Here's how the part is built. I have some questions about the finished solid (model axes, mm). A direction names the side the tool comes from. Give positions to 0.01 mm unless a question says otherwise; leave off trailing zeros. Write each loop counter-clockwise with the first axis right and the second up, starting at its lowest first coordinate (ties: lowest second). Pieces come first, ordered by that corner, then holes. Notation, with made-up numbers: (65, 30) - (77, 30) arc R20 ccw to (77, 51) - close; hole circle Ø1 at (35.25, -15). An arc over 180 degrees is marked (long way). Use a Markdown table: item, result.
```python
from build123d import *

# Parameters (mm, degrees)
ESQUISSE1_R             = 15
BOSS_EXTRU_1_DEPTH      = 650
ESQUISSE2_R             = 15
ESQUISSE2_R_2           = 10
ENL_V_MAT_EXTRU_1_DEPTH = 60
ESQUISSE3_R             = 2
ENL_V_MAT_EXTRU_2_DEPTH = 50
D_GAGEMENT_M81_D        = 9
ESQUISSE6_R             = 0.5
ENL_V_MAT_EXTRU_3_DEPTH = 580
ENL_V_START             = -70
ESQUISSE7_R             = 15
ENL_V_MAT_EXTRU_4_DEPTH = 70


with BuildPart() as part:
    # Esquisse1 → Boss.-Extru.1 (new body)
    with BuildSketch(Plane(origin=(0, 0, 0), x_dir=(1, 0, 0), z_dir=(0, 1, 0))):
        with Locations(Location((0, 0, 0), (0, 0, 270))):
            Circle(ESQUISSE1_R)
    extrude(amount=BOSS_EXTRU_1_DEPTH)

    # Esquisse2 → Enlèv. mat.-Extru.1 (cut)
    with BuildSketch(Plane(origin=(0, 0, 0), x_dir=(-1, 0, 0), z_dir=(0, -1, 0))):
        with Locations(Location((0, 0, 0), (0, 0, 90))):
            Circle(ESQUISSE2_R)
        with Locations(Location((0, 0, 0), (0, 0, 90))):
            Circle(ESQUISSE2_R_2, mode=Mode.SUBTRACT)
    extrude(amount=-ENL_V_MAT_EXTRU_1_DEPTH, mode=Mode.SUBTRACT)

    # Esquisse3 → Enlèv. mat.-Extru.2 (cut)
    with BuildSketch(Plane(origin=(0, 0, 0), x_dir=(-1, 0, 0), z_dir=(0, -1, 0))):
        with Locations(Location((0, 0, 0), (0, 0, 90))):
            Circle(ESQUISSE3_R)
    extrude(amount=-ENL_V_MAT_EXTRU_2_DEPTH, mode=Mode.SUBTRACT)

    # Dégagement M81 (through all)
    with Locations(Plane(origin=(-15, 84, 0), x_dir=(0, 0, -1), z_dir=(-1, 0, 0))):
        with Locations((0, 0), (0, -480)):
            Hole(D_GAGEMENT_M81_D / 2)

    # Esquisse6 → Enlèv. mat.-Extru.3 (cut)
    with BuildSketch(Plane(origin=(0, 650, 0), x_dir=(1, 0, 0), z_dir=(0, 1, 0))):
        with Locations(Location((0, 0, 0), (0, 0, 270))):
            Circle(ESQUISSE6_R)
    extrude(amount=-ENL_V_MAT_EXTRU_3_DEPTH, mode=Mode.SUBTRACT)

    # Esquisse7 → Enlèv. mat.-Extru.4 (cut)
    with BuildSketch(Plane(origin=(0, 650, 0), x_dir=(1, 0, 0), z_dir=(0, 1, 0)).offset(ENL_V_START)):
        with Locations(Location((0, 0, 0), (0, 0, 90))):
            Circle(ESQUISSE7_R)
    extrude(amount=ENL_V_MAT_EXTRU_4_DEPTH, mode=Mode.SUBTRACT)


solid = part.part
```
Item 1: For faces 5 (the cylindrical face through (4.506, 316.36, 14.307)), 6 (the flat face through (-3, 60, -10)), which set-ups out of +Z, -Z, +X, -X, +Y, -Y let a thin tool reach every point of the face, with its end or its side?
Values:
| item | result |
|---|---|
| face 5 | +Y, -Y |
| face 6 | -Y |
Item 2: I need wall thicknesses on line 1 along Y through (x, z) = (13, 1); line 2 along X through (y, z) = (574.75, 0). Which ranges of each line are inside material? Lowest first, please. Write a range as [from, to].
Values:
| item | result |
|---|---|
| line 1 | y = [60, 79.61], [88.39, 559.61], [568.39, 580] |
| line 2 | x = [-15, -0.5], [0.5, 15] |
Item 3: Will these pins go through, and if not, where does the flat tip stop? pin 1 Ø8 at (x, y) = (1, 233.5) entering from +Z; pin 2 Ø4 at (x, z) = (-9, -11) entering from -Y; pin 3 Ø12 at (y, z) = (296, 8) entering from -X; pin 4 Ø8 at (x, y) = (-7.5, 197) entering from -Z.
Values:
| item | result |
|---|---|
| pin 1 | stops at z = 15 |
| pin 2 | stops at y = 60 |
| pin 3 | stops at x = -14.87 |
| pin 4 | stops at z = -14.59 |
Item 4: If we section it at A-A, the plane y = 387: Write out the boundary of the cut face in (x, z), plus the area to 3 significant figures.
Values:
| item | result |
|---|---|
| outline | circle Ø30 at (0, 0); hole circle Ø1 at (0, 0) |
| area | 706 mm2 |
Item 5: Thinking about a two-plate mould opening in Y: for faces 1 (the flat face through (0, 580, -3)), 2 (the cylindrical face through (0.21, 80.206, 2.419)), 3 (the flat face through (2.4, 0, -0.1)), 4 (the cylindrical face through (0.21, 560.206, 2.419)), which applies, +Y half, -Y half, draft (parallel to the pull), parting line (faces both ways), or undercut?
Values:
| item | result |
|---|---|
| face 1 | +Y half |
| face 2 | undercut |
| face 3 | -Y half |
| face 4 | undercut |
